Part print with two shaded views. Sizes in mm from the minimum x, y, z corner. A direction names the side the tool comes from. Give positions to 0.01 mm unless a question says otherwise; leave off trailing zeros. Write each loop counter-clockwise with the first axis right and the second up, starting at its lowest first coordinate (ties: lowest second). Pieces come first, ordered by that corner, then holes.
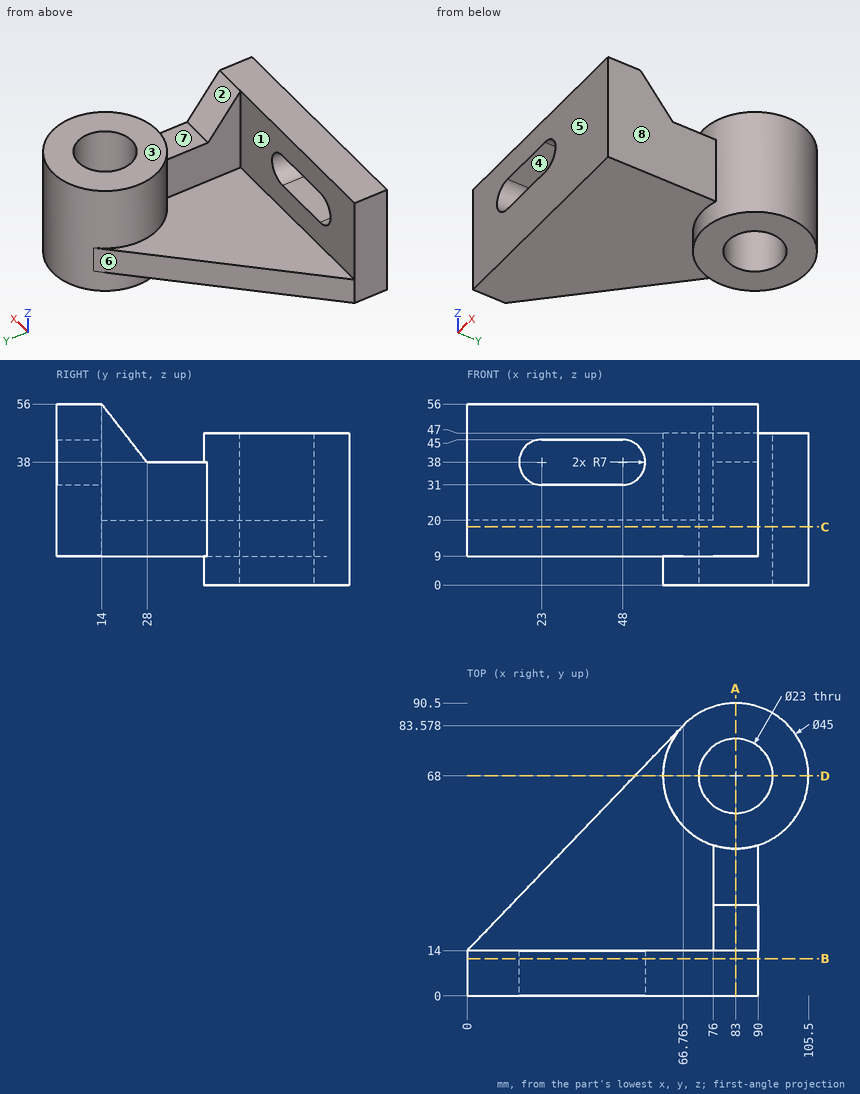
1) Saw through at C-C, the plane z = 18. Write the cut outline in (x, y) (1 decimal).
Answers follow:
outline: (0, 0) - (90, 0) - (90, 46.6) arc R22.5 ccw (long way) to (66.8, 83.6) - (0, 14) - close; hole circle Ø23 at (83, 68)
2) Saw through at B-B, the plane y = 11.5. Write the cut outline in (x, z).
Answers follow:
outline: (0, 9) - (90, 9) - (90, 56) - (0, 56) - close; hole (23, 31) - (48, 31) arc R7 ccw to (48, 45) - (23, 45) arc R7 ccw to start
3) Saw through at A-A, the plane x = 83. Write the cut outline in (y, z).
Answers follow:
outline: (0, 9) - (45.5, 9) - (45.5, 0) - (56.5, 0) - (56.5, 47) - (45.5, 47) - (45.5, 38) - (28, 38) - (14, 56) - (0, 56) - close; (79.5, 0) - (90.5, 0) - (90.5, 47) - (79.5, 47) - close
4) Pin check, flat tips, straight feed: pin 1 Ø1 at (y, z) = (62.5, 24) entering from -X; pin 2 Ø5 at (x, z) = (43, 24) entering from -Y; pin 3 Ø14 at (y, z) = (14.5, 39) entering from +X; pin 4 Ø10 at (x, z) = (75.5, 19.5) entering from +Y. Stop position of each tip, or through.
Answers follow:
pin 1: stops at x = 61.06
pin 2: stops at y = 0
pin 3: stops at x = 90
pin 4: stops at y = 90.36
5) Wall check: L1, parallel to Y at x = 83, z = 20; L2, parallel to X at y = 19.5, z = 29.5; L3, parallel to Z at x = 33, y = 29.5. Give the ranges that are in metal, low to high.
Answers follow:
L1: y = 0 to 56.5, 79.5 to 90.5
L2: x = 76 to 90
L3: z = 9 to 20
6) 3-axis set-ups, long thin cutter, end or side, ignore diameter. For the marked faces 1, 2, 3 and 4: which of +Z, -Z, +X, -X, +Y, -Y reach the whole face in a straight line?
Answers follow:
face 1: +Z, -X
face 2: +Z, +X, -X
face 3: +Z, +X, -X, +Y
face 4: +Y, -Y
7) Two-plate mould, pull along Y, no slides. Class the marked faces 5, 6, 7 and 8: +Y half, -Y half, draft (parallel to the pull), parting line (faces both ways), or undercut.
Answers follow:
face 5: -Y half
face 6: +Y half
face 7: undercut
face 8: draft
8) Saw through at D-D, the plane y = 68. Write the cut outline in (x, z).
Answers follow:
outline: (51.82, 9) - (60.5, 9) - (60.5, 0) - (71.5, 0) - (71.5, 47) - (60.5, 47) - (60.5, 20) - (51.82, 20) - close; (94.5, 0) - (105.5, 0) - (105.5, 47) - (94.5, 47) - close
